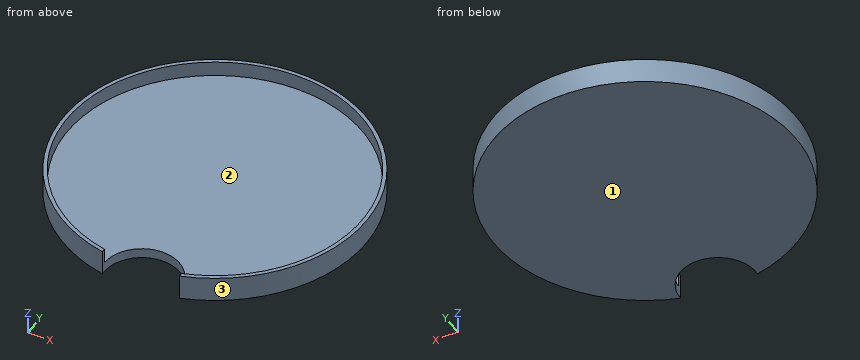
Autodesk Fusion 360 part; units mm, degrees
sketch "Sketch1" plane through (0, 0, 0) normal (0, 0, 1) x (1, 0, 0)
  circle A0 centre (0, 0) radius 77.5
  dimension "d1" = 155
sketch "Sketch2" plane through (0, 0, 0) normal (0, 0, 1) x (1, 0, 0)
  circle A0 centre (0, 0) radius 60
  dimension "d4" = 120
extrude "Extrude2" add sketch "Sketch2" along normal blind 10
hole "Hole1" at (3.3713, -57.3197, 10) direction (0, 0, -1) diameter 30 end through all
hole "Hole2" at (0, 0, 10) direction (0, 0, -1) diameter 117 depth 6 tip angle 180
Could you check a few things on this model? Use its own coordinates, in mm. Face numbers are marked on the shaded views. Give positions to 0.01 mm unless a question says otherwise; leave off trailing zeros. Write each loop counter-clockwise with the first axis right and the second up, starting at its lowest first coordinate (ties: lowest second). Pieces come first, ordered by that corner, then holes. Notation, with made-up numbers: (50.25, 37.5) - (62.25, 37.5) arc R28 cw to (62.25, 65.5) - close; hole circle Ø5 at (-2, 71). An arc over 180 degrees is marked (long way). Use CSV: the item, a comma, the result in double quotes. Start each with the question number.
Item 1: I want a section at A-A, the plane y = 0. Please give me the cut outline in (x, z), then the cut area to 3 significant figures.
Item 2: If we mould it in two halves opening along X, with no side actions, what happens to the marked faces 1, 2 and 3? For each: pulls with the +X half, pulls with the -X half, needs draft (parallel to the pull), parting line crosses it, or undercut.
Item 3: I want a section at B-B, the plane x = -17.5. Please give me the cut outline in (y, z).
Item 4: I want a section at D-D, the plane x = 0. Please give me the cut outline in (y, z).
Item 5: I'm going to push flat-ended pins straight in: pin 1 (4 mm diameter, centred on x = -5.5, y = 3, fed in from +Z); pin 2 (3 mm diameter, centred on x = 44.5, z = 2, fed in from -Y); pin 3 (3 mm diameter, centred on y = 40.5, z = 3, fed in from -X). Where does each tip first touch, or does it pass through?
Item 6: If I drill on line 1 along X through (y, z) = (0, 8.3); line 2 along Y through (x, z) = (0, 8.2); line 3 along Z through (x, y) = (-1, -12), over which ranges is the centre line in solid material (lowest first)?
Item 7: I want a section at C-C, the plane z = 7.5. Please give me the cut outline in (x, y), then the cut area to 3 significant figures.
Findings:
1,outline,"(-60, 0) - (60, 0) - (60, 10) - (58.5, 10) - (58.5, 4) - (-58.5, 4) - (-58.5, 10) - (-60, 10) - close"
1,area,"498 mm2"
2,face 1,"needs draft"
2,face 2,"undercut"
2,face 3,"parting line crosses it"
3,outline,"(-57.39, 0) - (57.39, 0) - (57.39, 10) - (55.82, 10) - (55.82, 4) - (-55.82, 4) - (-55.82, 10) - (-57.39, 10) - close"
4,outline,"(-42.7, 0) - (60, 0) - (60, 10) - (58.5, 10) - (58.5, 4) - (-42.7, 4) - close"
5,pin 1,"stops at z = 4"
5,pin 2,"stops at y = -41.84"
5,pin 3,"stops at x = -45.6"
6,line 1,"x = -60 to -58.5, 58.5 to 60"
6,line 2,"y = 58.5 to 60"
6,line 3,"z = 0 to 4"
7,outline,"(-11.63, -57.33) arc R58.5 cw (long way) to (18.27, -55.57) arc R15 cw to (18.37, -57.12) arc R60 ccw (long way) to (-11.55, -58.88) arc R15 cw to start"
7,area,"513 mm2"
